Here's how the part is built. I have some questions about the finished solid (model axes, mm). Face numbers are marked on the shaded views. A direction names the side the tool comes from. Give positions to 0.01 mm unless a question says otherwise; leave off trailing zeros. Order: outer loops, then holes, each group sorted by start corner. A loop starts at its lowest first (then second) coordinate and runs counter-clockwise, first axis right, second up.
Autodesk Inventor part; units mm, degrees
ref_plane "YZ Plane" through (0, 0, 0) normal (1, 0, 0) x (0, 1, 0)
ref_plane "XZ Plane" through (0, 0, 0) normal (0, 1, 0) x (-1, 0, 0)
ref_plane "XY Plane" through (0, 0, 0) normal (0, 0, 1) x (1, 0, 0)
ref_plane "РабПлоскость1" through (57.3886, 15.9976, 24.7396) normal (1, 0, 0) x (0, 1, 0)
sketch "Эскиз1" plane through (57.3886, 15.9976, 24.7396) normal (1, 0, 0) x (0, 1, 0)
  circle A0 centre (-16.5, 48) radius 1.5
  circle A1 centre (-16.5, 31) radius 1.5
  circle A2 centre (-16.5, 40) radius 4
  circle A3 centre (-16.5, 40) radius 12.75
  circle A4 centre (-16.5, 132) radius 1.5
  circle A5 centre (-16.5, 115) radius 1.5
  circle A6 centre (-16.5, 124) radius 4
  circle A7 centre (-16.5, 124) radius 12.75
  line L0 (-3.75, 40) -> (-2.75, 40)
  line L1 (-30.75, 6.25) -> (-30.75, 157.25)
  line L2 (-30.75, 157.25) -> (-2.75, 157.25)
  line L3 (-30.75, 6.25) -> (0.25, 6.25)
  line L4 (0.25, 6.25) -> (0.25, 157.25)
  line L5 (0.25, 157.25) -> (-30.75, 157.25)
  line L6 (-30.75, 157.25) -> (-30.75, 6.25)
  point P0 (-15.9976, -24.7396)
  point P1 (-15.5, 28.25)
  point P2 (-2.75, 157.25)
  dimension "d15" = 25.5
  dimension "d43" = 25.5
  dimension "d44" = 1
  dimension "d45" = 28
  dimension "d46" = 151
  dimension "d79" = 31
ref_plane "РабПлоскость2" through (57.3886, 13.2476, 181.9896) normal (0, 1, 0) x (1, 0, 0)
sketch "Эскиз5" plane through (57.3886, 13.2476, 181.9896) normal (0, 1, 0) x (1, 0, 0)
  line L0 (-3, 0) -> (-23, 0)
  line L1 (-23, 0) -> (-23, 20)
  line L2 (-3, 20) -> (-3, 0)
  line L3 (-3, 151) -> (-3, 0)
  line L4 (-23, 0) -> (-3, 0)
  line L5 (-3, 0) -> (-3, 5)
  line L6 (-23, 5) -> (-23, 0)
  line L7 (-23, 0) -> (-18, 0)
  line L8 (-23, 20) -> (-23, 0)
  line L9 (-3, 20) -> (-3, 15)
  line L10 (-23, 15) -> (-23, 20)
  line L11 (-8, 0) -> (-3, 0)
  line L12 (-3, 0) -> (-3, 20)
  circle A0 centre (-18, 5) radius 1.5
  circle A1 centre (-18, 15) radius 1.5
  circle A2 centre (-8, 15) radius 1.5
  circle A3 centre (-8, 5) radius 1.5
  line L13 (-3, 151) -> (-23, 151)
  line L14 (-23, 151) -> (-23, 131)
  line L15 (-3, 131) -> (-3, 151)
  line L16 (-3, 151) -> (-23, 151)
  line L17 (-23, 151) -> (-23, 146)
  line L18 (-3, 146) -> (-3, 151)
  line L19 (-23, 151) -> (-18, 151)
  line L20 (-23, 131) -> (-23, 151)
  line L21 (-3, 131) -> (-3, 136)
  line L22 (-23, 136) -> (-23, 131)
  line L23 (-8, 151) -> (-3, 151)
  line L24 (-3, 151) -> (-3, 131)
  circle A4 centre (-18, 136) radius 1.5
  circle A5 centre (-18, 146) radius 1.5
  circle A6 centre (-8, 146) radius 1.5
  circle A7 centre (-8, 136) radius 1.5
  line L25 (-23, 20) -> (-23, 131)
  line L26 (-3, 20) -> (-3, 131)
  point P0 (-57.3886, 181.9896)
  point P1 (-23, 131)
ref_plane "РабПлоскость3" through (57.3886, -14.7524, 181.9896) normal (0, 0, 1) x (1, 0, 0)
sketch "Эскиз6" plane through (57.3886, -14.7524, 181.9896) normal (0, 0, 1) x (1, 0, 0)
  line L0 (-3, 28) -> (-23, 28)
  line L1 (-3, 25) -> (-23, 25)
  line L2 (-23, 28) -> (-23, 25)
  line L3 (0, 0) -> (-3, 0)
  line L4 (-23, 25) -> (-3, 0)
  line L5 (-3, 0) -> (0, 0)
  line L6 (0, 28) -> (0, 0)
  line L7 (0, 0) -> (0, 28)
  line L8 (0, 28) -> (-23, 28)
  point P0 (-57.3886, 14.7524)
ref_plane "РабПлоскость4" through (57.3886, -14.7524, 30.9896) normal (0, 0, -1) x (-1, 0, 0)
sketch "Эскиз7" plane through (57.3886, -14.7524, 30.9896) normal (0, 0, -1) x (-1, 0, 0)
  line L0 (0, 28) -> (0, 0)
  line L1 (3, 28) -> (23, 28)
  line L2 (0, 28) -> (23, 28)
  line L3 (3, 25) -> (23, 25)
  line L4 (23, 28) -> (23, 25)
  line L5 (0, 0) -> (3, 0)
  line L6 (23, 25) -> (3, 0)
  line L7 (3, 0) -> (0, 0)
  line L8 (0, 0) -> (0, 28)
  point P0 (57.3886, 14.7524)
extrude "Выдавливание8" add sketch "Эскиз7" along normal blind 3
extrude "Выдавливание9" add sketch "Эскиз6" along normal blind 3
extrude "Выдавливание10" add sketch "Эскиз1" against normal blind 3 contours A3 | A7 | L1 L2 L5 L4 L3
extrude "Выдавливание11" add sketch "Эскиз5" along normal blind 3
sketch "Эскиз8" plane through (57.3886, 16.2476, 181.9896) normal (0, 1, 0) x (1, 0, 0)
  line L0 (0, 151) -> (0, 154)
  line L1 (-23, 154) -> (0, 154)
  line L2 (0, 151) -> (-23, 151)
  line L3 (-23, 151) -> (-23, 154)
  line L4 (-23, 154) -> (0, 154)
  line L5 (0, 154) -> (0, 151)
  line L6 (0, 0) -> (0, -3)
  line L7 (0, -3) -> (-23, -3)
  line L8 (0, 0) -> (-23, 0)
  line L9 (-23, 0) -> (-23, -3)
  line L10 (-23, -3) -> (0, -3)
  line L11 (0, -3) -> (0, 0)
  point P0 (-57.3886, 181.9896)
extrude "Выдавливание12" add sketch "Эскиз8" against normal blind 3
fillet "Сопряжение7" radius 1 1 edges at (57.3886, -14.7524, 106.4896)
fillet "Сопряжение8" radius 1 1 edges at (54.3886, -14.7524, 106.4896)
fillet "Сопряжение9" radius 2 1 edges at (54.3886, -14.7524, 183.4896)
fillet "Сопряжение10" radius 2 1 edges at (54.3886, -14.7524, 29.4896)
properties part number "крепёж_мотора_f"
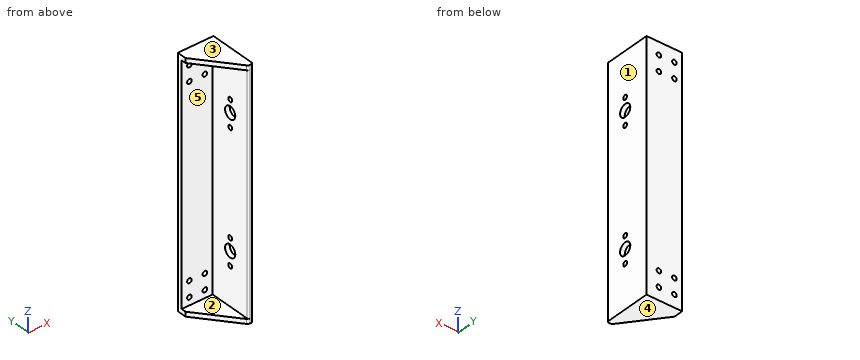
Q1. If we section it at A-A on z = 89: List the corners of the cut face in (x, y) for me, plus the area to 3 significant figures.
Filled sheet:
outline: (34.39, 13.25) - (54.39, 13.25) - (54.39, -13.75) arc R1 ccw to (55.39, -14.75) - (56.39, -14.75) arc R1 ccw to (57.39, -13.75) - (57.39, 16.25) - (34.39, 16.25) - close
area: 153 mm2
Q2. For the marked faces 1 and 2, which set-ups out of +Z, -Z, +X, -X, +Y, -Y let a thin tool reach every point of the face, with its end or its side?
Filled sheet:
face 1: +Z, -Z, +X, +Y, -Y
face 2: -X, -Y
Q3. I'm going to push flat-ended pins straight in: P1, Ø4, axis at y = -0.5, z = 72.74, coming from the -X side; P2, Ø6, axis at x = 49, z = 109, coming from the -Y side. Where does each tip first touch, or does it pass through?
Filled sheet:
P1: stops at x = 54.39
P2: stops at y = 13.25
Q4. If we section it at B-B on x = 45.25: List the corners of the cut face in (y, z) for me.
Filled sheet:
outline: (-3.33, 27.99) - (16.25, 27.99) - (16.25, 184.99) - (-3.33, 184.99) - (-3.33, 181.99) - (13.25, 181.99) - (13.25, 30.99) - (-3.33, 30.99) - close
Q5. I need wall thicknesses on L1, parallel to Z at x = 50.5, y = -5.5; L2, parallel to Y at x = 52.5, z = 163.5; L3, parallel to X at y = 9, z = 57.5. Which ranges of each line are inside material? Lowest first, please.
Filled sheet:
L1: z = 27.99 to 30.99, 181.99 to 184.99
L2: y = 13.25 to 16.25
L3: x = 54.39 to 57.39
Q6. Thinking about a two-plate mould opening in Z: for the marked faces 3, 4 and 5, which applies, released by +Z, released by -Z, zero draft, split by the parting line, or undercut?
Filled sheet:
face 3: released by +Z
face 4: released by -Z
face 5: undercut
